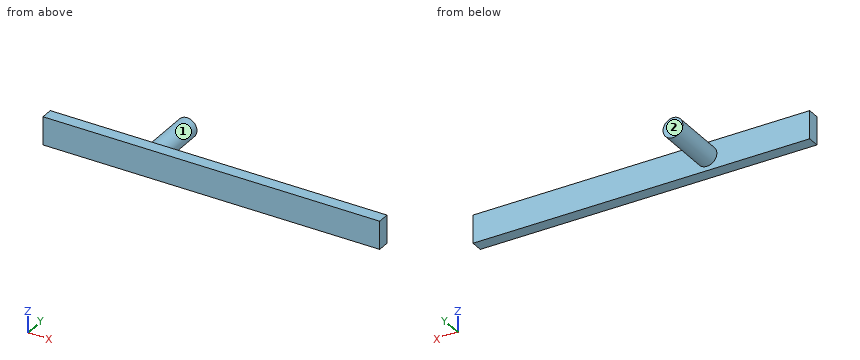
```python
from build123d import *

# Parameters (mm, degrees)
SKETCH1_W           = 1066.8
SKETCH1_H           = 88.9
BOSS_EXTRUDE1_DEPTH = 38.1
SKETCH2_R           = 31.428028039
BOSS_EXTRUDE2_DEPTH = 177.8


with BuildPart() as part:
    # Sketch1 → Boss-Extrude1 (new body)
    with BuildSketch(Plane(origin=(0, 0, 0), x_dir=(1, 0, 0), z_dir=(0, 1, 0))):
        with Locations((533.4, 44.45)):
            Rectangle(SKETCH1_W, SKETCH1_H)
    extrude(amount=BOSS_EXTRUDE1_DEPTH)

    # Sketch2 → Boss-Extrude2 (add)
    with BuildSketch(Plane(origin=(0, 38.1, 0), x_dir=(1, 0, 0), z_dir=(0, 1, 0))):
        with Locations((325.671457389, 43.854789276)):
            Circle(SKETCH2_R)
    extrude(amount=BOSS_EXTRUDE2_DEPTH)


solid = part.part
```
Check sheet for the modelled part. Datum: model origin and axes. Units: mm. Face numbers are marked on the shaded views. A direction names the side the tool comes from. Give positions to 0.01 mm unless a question says otherwise; leave off trailing zeros. Write each loop counter-clockwise with the first axis right and the second up, starting at its lowest first coordinate (ties: lowest second). Pieces come first, ordered by that corner, then holes.
Item 1: Gauge pin test, flat ends, axial feed: pin 1 (6 mm diameter, centred on y = 45, z = -64.5, fed in from -X); pin 2 (3 mm diameter, centred on y = 192, z = -57, fed in from -X); pin 3 (1.5 mm diameter, centred on y = 82, z = -18, fed in from -X). Record the tip position at first contact, or that the pin passes through.
Item 2: Access from +Z, -Z, +X, -X, +Y, -Y to the whole of each face (thin tool, end or side, straight path). Record for the marked faces 1 and 2.
Item 3: Cross-section at A-A (z = -53). Enter the section's corners in (x, y), and give its area (3 significant figures).
Item 4: Cross-section at D-D (y = 134.5). Enter the section's corners in (x, z).
Item 5: Cross-section at B-B (x = 483). Enter the section's corners in (y, z).
Item 6: Scan lines: L1, parallel to Y at x = 849, z = -72; L2, parallel to X at y = 155, z = -29; L3, parallel to X at y = 164.5, z = -52. Record each from-to range of solid material in increasing order.
Item 7: Cross-section at C-C (x = 337.5). Enter the section's corners in (y, z), and give its area (3 significant figures).
Report:
1. pin 1: stops at x = 299.66
1. pin 2: stops at x = 296.48
1. pin 3: stops at x = 306.76
2. face 1: +Y
2. face 2: +Z, -Z, +X, -X, +Y
3. outline: (0, 0) - (1066.8, 0) - (1066.8, 38.1) - (355.74, 38.1) - (355.74, 215.9) - (295.6, 215.9) - (295.6, 38.1) - (0, 38.1) - close
3. area: 51,300 mm2
4. outline: circle Ø62.86 at (325.67, -43.85)
5. outline: (0, -88.9) - (38.1, -88.9) - (38.1, 0) - (0, 0) - close
6. L1: y = 0 to 38.1
6. L2: x = 297.98 to 353.37
6. L3: x = 295.32 to 356.03
7. outline: (0, -88.9) - (38.1, -88.9) - (38.1, -72.97) - (215.9, -72.97) - (215.9, -14.74) - (38.1, -14.74) - (38.1, 0) - (0, 0) - close
7. area: 13,700 mm2
